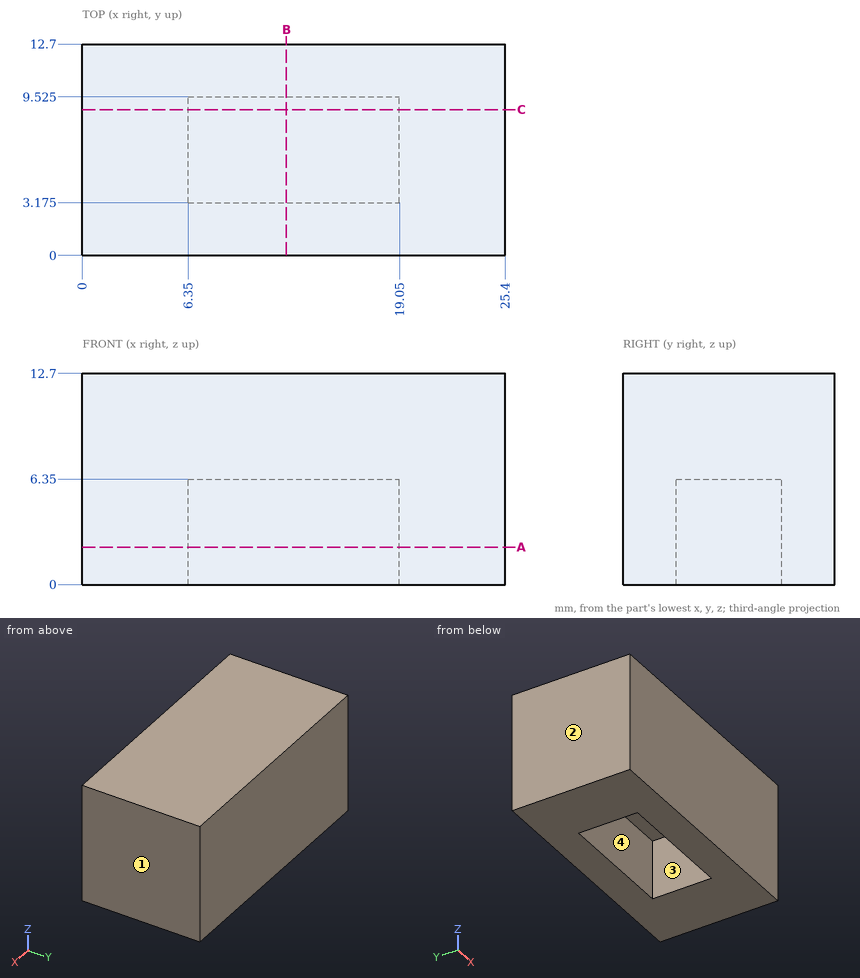
Input: dimensioned drawing with shaded views. Units: mm. Origin: part minimum x, y, z. Coordinates: 2 decimals unless noted, no trailing zeros. Write each loop counter-clockwise with the first axis right and the second up, starting at its lowest first coordinate (ties: lowest second). Pieces come first, ordered by that corner, then holes. Notation, with made-up numbers: M -19.75,-31.75 L -11.75,-31.75 A20 cw -11.75,-17.75 Z; hole C -2,61.5 d5. An arc over 180 degrees is marked long. Use one line per item in the form item = value.
Q1. Section A-A (z = 2.25). Return loops of the section in (x, y) (3 decimals), plus the area to 3 significant figures.
Answer below:
outline = M 0,0 L 25.4,0 L 25.4,12.7 L 0,12.7 Z; hole M 6.35,3.175 L 19.05,3.175 L 19.05,9.525 L 6.35,9.525 Z
area = 242 mm²
Q2. Section B-B (x = 12.25). Return loops of the section in (y, z) (3 decimals).
Answer below:
outline = M 0,0 L 3.175,0 L 3.175,6.35 L 9.525,6.35 L 9.525,0 L 12.7,0 L 12.7,12.7 L 0,12.7 Z
Q3. First-contact query: pin 1 (1.9 mm diameter, centred on x = 11, z = 1.5, fed in from -Y); pin 2 (1.5 mm diameter, centred on x = 17, y = 4.5, fed in from -Z). Flat tips, straight axial feed; report the tip coordinate or a pass-through.
Answer below:
pin_1 = 0
pin_2 = 6.35
Q4. Draft query along X for the marked faces 1, 2, 3 and 4. Return one class per face: released by +X, released by -X, zero draft, split by the parting line, or undercut.
Answer below:
face_1 = released by +X
face_2 = released by -X
face_3 = undercut
face_4 = undercut
Q5. Section C-C (y = 8.75). Return loops of the section in (x, z).
Answer below:
outline = M 0,0 L 6.35,0 L 6.35,6.35 L 19.05,6.35 L 19.05,0 L 25.4,0 L 25.4,12.7 L 0,12.7 Z
Q6. Material intervals for probe 1 along X at (y, z) = (4, 4.75); probe 2 along Z at (x, y) = (18.75, 4), sorted ascending. Write a range as from..to.
Answer below:
probe_1 = 0..6.35, 19.05..25.4
probe_2 = 6.35..12.7
